```python
from build123d import *


# Not quite as in the source:
# - a fillet or chamfer that OpenCascade refuses, or shapes differently, is made with other operations: its cross-section is extruded or revolved along the edge and cut away or added


with BuildPart() as f1:
    # F0 (on Right) → F1 (revolve)
    with BuildSketch(Plane.YZ):
        Polygon((0, -5), (0, -2.5), (-8, -2.5), (-8, -4.5), (-6, -6.25), (-5, -5), align=None)
    revolve(axis=Axis((0, -4, 0), (0, -1, 0)))

    # F2: chamfer of 0.25 on 4 edges, made by hand

    # F2_s1 → F2_t2 (revolve)
    with BuildSketch(Plane.YZ):
        Polygon((-5.0750609905, -5.0938262381), (-4.8798437881, -5), (-5, -5), align=None)
    revolve(axis=Axis((0, -5, 0), (0, -1, 0)))

    # F2_s3 → F2_t4 (revolve, cut)
    with BuildSketch(Plane.YZ):
        Polygon((-7.75, -2.5), (-8, -2.75), (-8, -2.5), align=None)
    revolve(axis=Axis((0, -8, 0), (0, -1, 0)), mode=Mode.SUBTRACT)

    # F2_s5 → F2_t6 (revolve, cut)
    with BuildSketch(Plane.YZ):
        Polygon((0, -2.75), (-0.25, -2.5), (0, -2.5), align=None)
    revolve(axis=Axis((0, 0, 0), (0, -1, 0)), mode=Mode.SUBTRACT)

    # F2_s7 → F2_t8 (revolve, cut)
    with BuildSketch(Plane.YZ):
        Polygon((0, -4.75), (-0.25, -5), (0, -5), align=None)
    revolve(axis=Axis((0, 0, 0), (0, -1, 0)), mode=Mode.SUBTRACT)


solid = f1.part
```
Read the model definition and answer for the solid it produces. Units are mm, in the model's axes. Coordinates: 2 decimals unless noted, no trailing zeros. Write each loop counter-clockwise with the first axis right and the second up, starting at its lowest first coordinate (ties: lowest second). Pieces come first, ordered by that corner, then holes. Notation, with made-up numbers: (15.25, -29.75) - (60.25, -29.75) arc R20 cw to (60.25, 9.25) - close; hole circle Ø11 at (-2, 36). An arc over 180 degrees is marked (long way). Answer as a JSON object with one key per item and string values. Group by question number.
1. A cutting plane is placed at D-D (y = -5.5). Determine the outline of the cut face in (x, z) (3 decimals), plus the area to 3 significant figures.
2. Consider L1, parallel to X at y = -3.5, z = 0; L2, parallel to Z at x = 1.5, y = -1; L3, parallel to X at y = -7, z = 1. Determine where each line is inside the solid, lowest interval first. Write a range as [from, to].
3. A cutting plane is placed at B-B (x = 0). Determine the outline of the cut face in (y, z).
4. A cutting plane is placed at A-A (z = 0). Determine the outline of the cut face in (x, y), plus the area to 3 significant figures.
5. Each of these flat-tipped pins is pushed along its axis until it touches: P1, Ø1, axis at y = -5, z = -4, coming from the +X side; P2, Ø2, axis at x = -4.5, y = -3, coming from the -Z side. Where does it stop, or does it pass through?
6. A cutting plane is placed at C-C (y = -4). Determine the outline of the cut face in (x, z), plus the area to 3 significant figures.
7. The mould has two halves that part along X. Classify faces 1 (the flat face through (-3, -8, 0)), 2 (the cylindrical face through (-2.44, -4.05, 0.54)), 3 (the cylindrical face through (-4.88, -2.53, 1.08)): +X half, -X half, draft (parallel to the pull), parting line (faces both ways), or undercut.
Worked out:
{
 "1": {"outline": "circle Ø11.25 at (0, 0); hole circle Ø5 at (0, 0)", "area": "79.8 mm²"},
 "2": {"L1": "x = [-5, -2.5], [2.5, 5]", "L2": "z = [-4.77, -2], [2, 4.77]", "L3": "x = [-5.28, -2.29], [2.29, 5.28]"},
 "3": {"outline": "(-8, -4.5) - (-6, -6.25) - (-5.08, -5.09) - (-4.88, -5) - (-0.25, -5) - (0, -4.75) - (0, -2.75) - (-0.25, -2.5) - (-7.75, -2.5) - (-8, -2.75) - close; (-8, 2.75) - (-7.75, 2.5) - (-0.25, 2.5) - (0, 2.75) - (0, 4.75) - (-0.25, 5) - (-4.88, 5) - (-5.08, 5.09) - (-6, 6.25) - (-8, 4.5) - close"},
 "4": {"outline": "(-6.25, -6) - (-4.5, -8) - (-2.75, -8) - (-2.5, -7.75) - (-2.5, -0.25) - (-2.75, 0) - (-4.75, 0) - (-5, -0.25) - (-5, -4.88) - (-5.09, -5.08) - close; (2.5, -7.75) - (2.75, -8) - (4.5, -8) - (6.25, -6) - (5.09, -5.08) - (5, -4.88) - (5, -0.25) - (4.75, 0) - (2.75, 0) - (2.5, -0.25) - close", "area": "42.6 mm²"},
 "5": {"P1": "stops at x = 4.08", "P2": "stops at z = -3.57"},
 "6": {"outline": "circle Ø10 at (0, 0); hole circle Ø5 at (0, 0)", "area": "58.9 mm²"},
 "7": {"face 1": "draft", "face 2": "undercut", "face 3": "parting line"}
}
